Build history of the part. All positions in model axes, mm. A direction names the side the tool comes from. Round coordinates to 2 decimals unless told otherwise and drop trailing zeros. Order: outer loops, then holes, each group sorted by start corner. A loop starts at its lowest first (then second) coordinate and runs counter-clockwise, first axis right, second up. Notation, with made-up numbers: (-40, 34.25) -> (5, 34.25) arc R18 cw to (5, 48.25) -> close; hole circle Ø10 at (57, -16). An arc over 180 degrees is marked (long way). Answer as a JSON object with one key per item and string values.
from build123d import *

# Parameters (mm, degrees)
BOSS_EXTRUDE1_DEPTH      = 190.5
BOSS_EXTRUDE1_DEPTH_BACK = 190.5
SKETCH2_W                = 381
SKETCH2_H                = 6.35
BOSS_EXTRUDE2_DEPTH      = 25.4
SKETCH3_R                = 3.96875
CUT_EXTRUDE1_DEPTH       = 25.4
SKETCH4_R                = 3.937
CUT_EXTRUDE2_DEPTH       = 302.34078715


with BuildPart() as part:
    # Sketch1 → Boss-Extrude1 (new, two sides: drawn at the far end of the back side and taken through both)
    with BuildSketch(Plane(origin=(0, 0, 0), x_dir=(0, 0, -1), z_dir=(1, 0, 0)).offset(-BOSS_EXTRUDE1_DEPTH_BACK)):
        with BuildLine():
            Line((-139.7, 0), (139.7, 0))
            ThreePointArc((139.7, 0), (193.581536726, 22.318463274), (215.9, 76.2))
            Line((215.9, 76.2), (203.2, 76.2))
            ThreePointArc((203.2, 76.2), (184.601280605, 31.298719395), (139.7, 12.7))
            Line((139.7, 12.7), (-139.7, 12.7))
            Line((-139.7, 12.7), (-139.7, 0))
        make_face()
    extrude(amount=BOSS_EXTRUDE1_DEPTH + BOSS_EXTRUDE1_DEPTH_BACK)

    # Sketch2 → Boss-Extrude2 (add)
    with BuildSketch(Plane(origin=(0, 76.2, 0), x_dir=(1, 0, 0), z_dir=(0, 1, 0))):
        with Locations((0, 206.375)):
            Rectangle(SKETCH2_W, SKETCH2_H)
    extrude(amount=BOSS_EXTRUDE2_DEPTH)

    # Sketch3 → Cut-Extrude1 (cut)
    with BuildSketch(Plane(origin=(0, 0, -209.55), x_dir=(-1, 0, 0), z_dir=(0, 0, -1))):
        with Locations((-139.7, 88.9)):
            Circle(SKETCH3_R)
        with Locations((139.7, 88.9)):
            Circle(SKETCH3_R)
        with Locations((0, 88.9)):
            Circle(SKETCH3_R)
    extrude(amount=-CUT_EXTRUDE1_DEPTH, mode=Mode.SUBTRACT)

    # Sketch4 → Cut-Extrude2 (cut, through all)
    with BuildSketch(Plane(origin=(0, 12.7, 0), x_dir=(1, 0, 0), z_dir=(0, 1, 0))):
        with Locations(Location((177.038, -119.888, 0), (0, 0, 270))):
            Circle(SKETCH4_R)
        with Locations(Location((177.038, 114.3, 0), (0, 0, 270))):
            Circle(SKETCH4_R)
        with Locations(Location((-177.038, -119.888, 0), (0, 0, 90))):
            Circle(SKETCH4_R)
        with Locations(Location((-177.038, 114.3, 0), (0, 0, 90))):
            Circle(SKETCH4_R)
        with Locations(Location((147.066, -2.794, 0), (0, 0, 270))):
            Circle(SKETCH4_R)
        with Locations(Location((-147.066, -2.794, 0), (0, 0, 270))):
            Circle(SKETCH4_R)
        with Locations(Location((121.666, -86.106, 0), (0, 0, 270))):
            Circle(SKETCH4_R)
    extrude(amount=-CUT_EXTRUDE2_DEPTH, mode=Mode.SUBTRACT)


solid = part.part
1) Cut at B-B, the plane z = -68.5. Give the cut face in (x, y), plus the area to 3 significant figures.
Checked values:
{"outline": "(-190.5, 0) -> (190.5, 0) -> (190.5, 12.7) -> (-190.5, 12.7) -> close", "area": "4,840 mm²"}
2) Probe L1, parallel to Y at x = 66, z = -2; L2, parallel to Z at x = 174, y = 82; L3, parallel to Z at x = 123, y = 68. List the from-to ranges inside material, lowest first. Write a range as from..to.
Checked values:
{"L1": "y = 0..12.7", "L2": "z = -209.55..-203.2", "L3": "z = -215.46..-202.67"}
3) Which spindle directions (+Z, -Z, +X, -X, +Y, -Y) get a long thin tool onto all of the face, cutting with end or side? Do faces 1 (the face through (-3, 86, -209.55)), 2 (the face through (-3, 12.7, -2)), 3 (the face through (-3, 0, 2)). Say none if no direction does.
Checked values:
{"face 1": "-Z, +X, -X, +Y", "face 2": "+Z, +X, -X, +Y", "face 3": "+Z, -Z, +X, -X, -Y"}
4) Cut at C-C, the plane y = 66. Give the cut face in (x, z), plus the area to 3 significant figures.
Checked values:
{"outline": "(-190.5, -215.21) -> (190.5, -215.21) -> (190.5, -202.38) -> (-190.5, -202.38) -> close", "area": "4,890 mm²"}
5) Flat gauge pins, fed straight in: pin 1 Ø1.5 at (x, z) = (148.5, -175.5) entering from +Y; pin 2 Ø7.5 at (x, y) = (0, 94.5) entering from +Z; pin 3 Ø1.9 at (x, z) = (54.5, -213.5) entering from +Y. Where does each tip first touch, or does it go through?
Checked values:
{"pin 1": "stops at y = 24.27", "pin 2": "stops at z = -203.2", "pin 3": "stops at y = 76.2"}
6) Cut at A-A, the plane x = 80. Give the cut face in (y, z).
Checked values:
{"outline": "(0, -139.7) arc R76.2 ccw to (76.2, -215.9) -> (76.2, -209.55) -> (101.6, -209.55) -> (101.6, -203.2) -> (76.2, -203.2) arc R63.5 cw to (12.7, -139.7) -> (12.7, 139.7) -> (0, 139.7) -> close"}
